from build123d import *

# Parameters (mm, degrees)
F0_R     = 30
F1_DEPTH = 60
F2_W     = 10
F2_H     = 20
F3_DEPTH = 50
F4_R     = 15
F5_DEPTH = 25
F6_R     = 10
F7_DEPTH = 100
F8_SIZE  = 4.99999


# Not quite as in the source:
# - a fillet or chamfer is up to 0.001 mm smaller than in the source, because OpenCascade refuses the exact size


with BuildPart() as f1:
    # F0 (on Top) → F1 (new body)
    with BuildSketch(Plane.XY):
        Circle(F0_R)
    extrude(amount=F1_DEPTH)

    # F2 (on Front) → F3 (cut, symmetric)
    with BuildSketch(Plane.XZ):
        with Locations((-25, 50)):
            Rectangle(F2_W, F2_H)
        with Locations((25, 50)):
            Rectangle(F2_W, F2_H)
    extrude(amount=F3_DEPTH, both=True, mode=Mode.SUBTRACT)

    # F4 (on face) → F5 (cut)
    with BuildSketch(Plane(origin=(0, 0, 0), x_dir=(1, 0, 0), z_dir=(0, 0, -1))):
        Circle(F4_R)
    extrude(amount=-F5_DEPTH, mode=Mode.SUBTRACT)

    # F6 (on face) → F7 (cut)
    with BuildSketch(Plane.XY.offset(60)):
        Circle(F6_R)
    extrude(amount=-F7_DEPTH, mode=Mode.SUBTRACT)

    # F8 (size 5 in the source; OpenCascade refuses exactly that, so slightly less here)
    f8_edges = [f1.edges().sort_by_distance(p)[0] for p in [
        (-10, 0, 25),
    ]]
    chamfer(f8_edges, length=F8_SIZE)


solid = f1.part
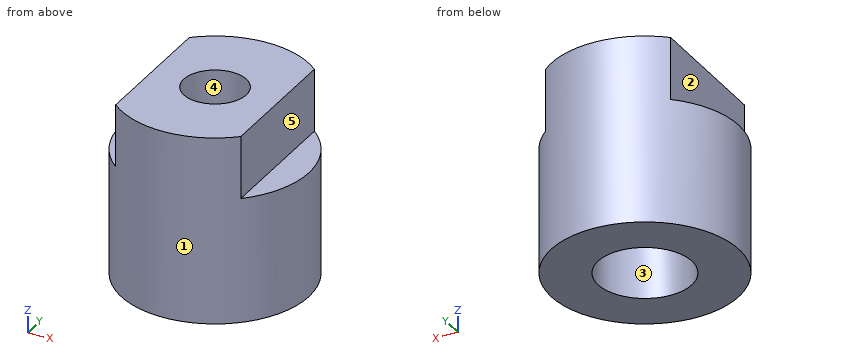
Verification items for the finished model (mm, model axes). Face numbers are marked on the shaded views. A direction names the side the tool comes from. Round coordinates to 2 decimals unless told otherwise and drop trailing zeros. Order: outer loops, then holes, each group sorted by start corner. A loop starts at its lowest first (then second) coordinate and runs counter-clockwise, first axis right, second up.
1. Thickness scan on L1, parallel to Y at x = 0, z = 18; L2, parallel to Y at x = 1, z = 38.5. Record the ranges inside material, lowest first.
Final values:
L1: y = -30 to -15, 15 to 30
L2: y = -29.98 to -9.95, 9.95 to 29.98
2. Section check D-D on y = 16.5. Record the cut outline in (x, z).
Final values:
outline: (-25.05, 0) - (25.05, 0) - (25.05, 40) - (20, 40) - (20, 60) - (-20, 60) - (-20, 40) - (-25.05, 40) - close
3. Section check C-C on z = 51. Record the cut outline in (x, y), then the cut area to 3 significant figures.
Final values:
outline: (-20, -22.36) arc R30 ccw to (20, -22.36) - (20, 22.36) arc R30 ccw to (-20, 22.36) - close; hole circle Ø20 at (0, 0)
area: 1,890 mm2
4. Release check for a two-part mould opening along Y. For the marked faces 1, 2 and 3 record: +Y half, -Y half, draft (parallel to the pull), parting line (faces both ways), or undercut.
Final values:
face 1: parting line
face 2: draft
face 3: undercut
5. Access from +Z, -Z, +X, -X, +Y, -Y to the whole of each face (thin tool, end or side, straight path). Record for the marked faces 4 and 5.
Final values:
face 4: +Z, -Z
face 5: +Z, +X, +Y, -Y
6. Go/stop test with flat-tipped pins: P1, Ø1, axis at y = 15, z = 14, coming from the +X side; P2, Ø8, axis at x = -5.5, z = 20.5, coming from the +Y side; P3, Ø8, axis at x = -24.5, y = 2.5, coming from the +Z side. Record where each tip stops, or that it passes through.
Final values:
P1: stops at x = 26.26
P2: stops at y = 29.96
P3: stops at z = 40
